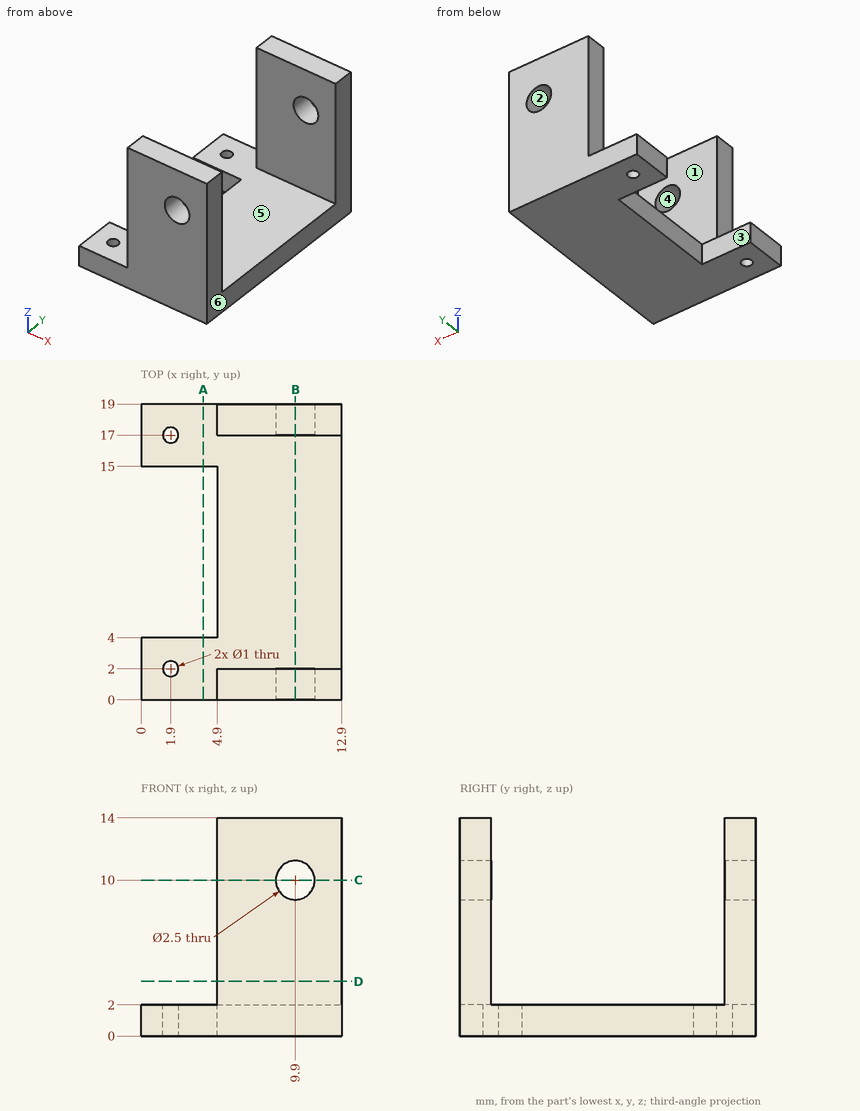
Drawing for the job (mm, zero at the part's lowest x, y, z). A direction names the side the tool comes from. Give positions to 0.01 mm unless a question says otherwise; leave off trailing zeros. Loops run counter-clockwise (first coordinate to the right, second up) from the corner with the lowest first, then second, coordinate; pieces in that order, holes last. Notation, with made-up numbers: (62, 4) - (82, 4) arc R17 ccw to (82, 14) - close; hole circle Ø1 at (-25.75, 20.5). An arc over 180 degrees is marked (long way). Write item = value, one per line. Start each with the question number.
1) Tool access for the marked faces 1, 2 and 3: list every direction of +Z, -Z, +X, -X, +Y, -Y with a clear straight run to the whole face (end or side of a thin tool).
2) Band-saw the part on B-B on x = 9.9. Give the cut face in (y, z).
3) Band-saw the part on D-D on z = 3.5. Give the cut face in (x, y), plus the area to 3 significant figures.
4) Drop flat-ended pins along their axis: pin 1 Ø4 at (x, y) = (7, 11.5) entering from +Z; pin 2 Ø2 at (y, z) = (1.5, 9) entering from -X. Give the stop position or say it passes through.
5) Probe probe 1 along Y at (x, z) = (1.9, 1.5); probe 2 along Y at (x, z) = (3, 1.25); probe 3 along Y at (x, z) = (10.5, 6). List the from-to ranges inside material, lowest first. Write a range as from..to.
6) Band-saw the part on A-A on x = 4. Give the cut face in (y, z).
7) Pull direction X, two halves, no side cores. Call the marked faces 4, 5 and 6: +X half, -X half, draft (parallel to the pull), parting line (faces both ways), or undercut.
8) Band-saw the part on C-C on z = 10. Give the cut face in (x, y).
Final values:
q1.face_1 = +Z, +X, -X
q1.face_2 = +Y, -Y
q1.face_3 = +Z, -Z, -X
q2.outline = (0, 0) - (19, 0) - (19, 8.75) - (17, 8.75) - (17, 2) - (2, 2) - (2, 8.75) - (0, 8.75) - close; (0, 11.25) - (2, 11.25) - (2, 14) - (0, 14) - close; (17, 11.25) - (19, 11.25) - (19, 14) - (17, 14) - close
q3.outline = (4.9, 0) - (12.9, 0) - (12.9, 2) - (4.9, 2) - close; (4.9, 17) - (12.9, 17) - (12.9, 19) - (4.9, 19) - close
q3.area = 32.0 mm²
q4.pin_1 = 2
q4.pin_2 = 4.9
q5.probe_1 = 0..1.5, 2.5..4, 15..16.5, 17.5..19
q5.probe_2 = 0..4, 15..19
q5.probe_3 = 0..2, 17..19
q6.outline = (0, 0) - (4, 0) - (4, 2) - (0, 2) - close; (15, 0) - (19, 0) - (19, 2) - (15, 2) - close
q7.face_4 = undercut
q7.face_5 = draft
q7.face_6 = +X half
q8.outline = (4.9, 0) - (8.65, 0) - (8.65, 2) - (4.9, 2) - close; (4.9, 17) - (8.65, 17) - (8.65, 19) - (4.9, 19) - close; (11.15, 0) - (12.9, 0) - (12.9, 2) - (11.15, 2) - close; (11.15, 17) - (12.9, 17) - (12.9, 19) - (11.15, 19) - close
